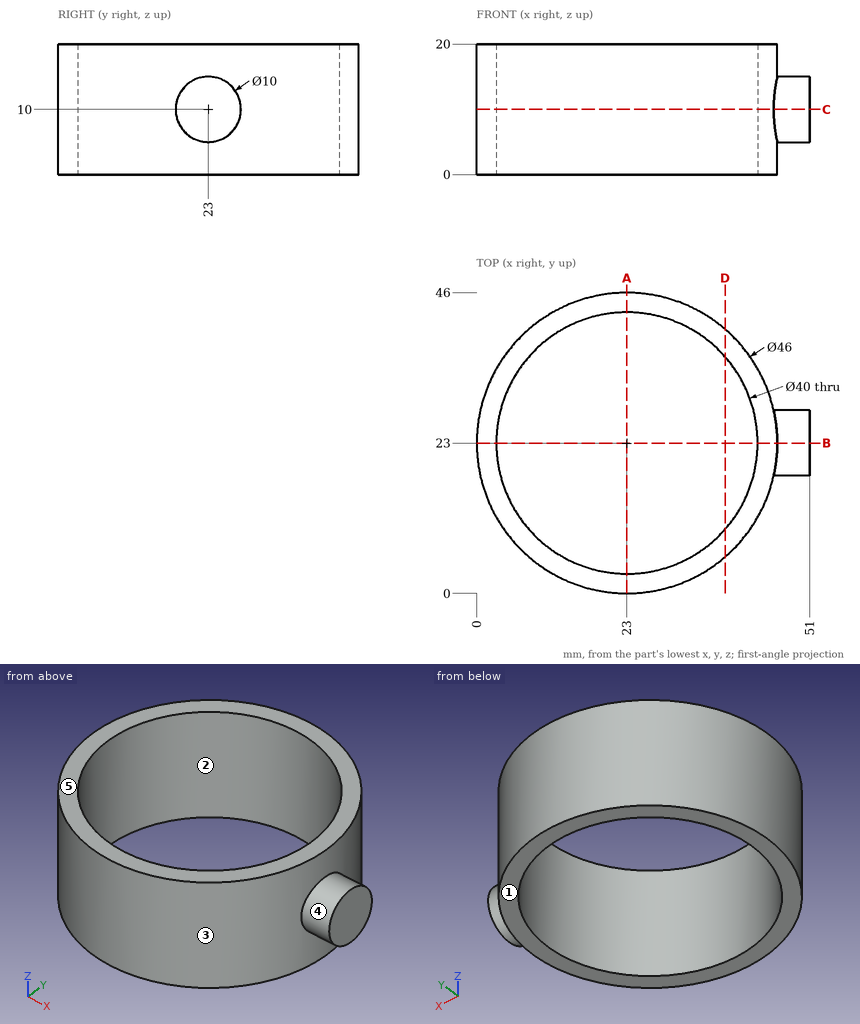
Can you work these out from the drawing? Everything is in mm from the part's minimum corner. A direction names the side the tool comes from. Coordinates: 2 decimals unless noted, no trailing zeros. Write each loop counter-clockwise with the first axis right and the second up, starting at its lowest first coordinate (ties: lowest second). Pieces come first, ordered by that corner, then holes. Notation, with made-up numbers: (75.5, 20) -> (117.5, 20) arc R27 ccw to (117.5, 59) -> close; hole circle Ø8 at (77.25, 15). An arc over 180 degrees is marked (long way). Write each question's results on one line, items separated by ' | '. Start each with the question number.
Q1. Imagine slicing it at D-D (x = 38). Write out the boundary of the cut face in (y, z).
Q2. We'd pull the mould along X, two halves only. Please class the marked faces 1, 2 and 3: +X half, -X half, draft (parallel to the pull), parting line (faces both ways), or undercut.
Q3. Imagine slicing it at C-C (z = 10). Write out the boundary of the cut face in (x, y), then the cut area to 3 significant figures.
Q4. On a 3-axis mill with a long thin cutter (end or side, diameter ignored), from which of +Z, -Z, +X, -X, +Y, -Y can I reach the whole of each face in a straight line? I mean the marked faces 4 and 5. Say none if no direction works.
Q5. Imagine slicing it at B-B (y = 23). Write out the boundary of the cut face in (x, z).
Q6. Imagine slicing it at A-A (x = 23). Write out the boundary of the cut face in (y, z), then the cut area to 3 significant figures.
Q7. I'm going to push flat-ended pins straight in: pin 1 (2 mm diameter, centred on x = 19.5, z = 7, fed in from +Y); pin 2 (6 mm diameter, centred on y = 27, z = 15.5, fed in from -X). Where does each tip first touch, or does it pass through?
Q8. If I drill on probe 1 along Y at (x, z) = (23, 10.5); probe 2 along X at (y, z) = (13, 11.5); probe 3 along Y at (x, z) = (21, 16.75), over which ranges is the centre line in solid material (lowest first)?
Taken from the geometry:
1) outline: (5.56, 0) -> (9.77, 0) -> (9.77, 20) -> (5.56, 20) -> close; (36.23, 0) -> (40.44, 0) -> (40.44, 20) -> (36.23, 20) -> close
2) face 1: draft | face 2: undercut | face 3: parting line
3) outline: (45.45, 18) -> (51, 18) -> (51, 28) -> (45.45, 28) arc R23 ccw (long way) to start; hole circle Ø40 at (23, 23) | area: 457 mm^2
4) face 4: +X | face 5: +Z, +X, -X, +Y, -Y
5) outline: (0, 0) -> (3, 0) -> (3, 20) -> (0, 20) -> close; (43, 0) -> (46, 0) -> (46, 5) -> (51, 5) -> (51, 15) -> (46, 15) -> (46, 20) -> (43, 20) -> close
6) outline: (0, 0) -> (3, 0) -> (3, 20) -> (0, 20) -> close; (43, 0) -> (46, 0) -> (46, 20) -> (43, 20) -> close | area: 120 mm^2
7) pin 1: stops at y = 45.86 | pin 2: stops at x = 0.02
8) probe 1: y = 0 to 3, 43 to 46 | probe 2: x = 2.29 to 5.68, 40.32 to 43.71 | probe 3: y = 0.09 to 3.1, 42.9 to 45.91
